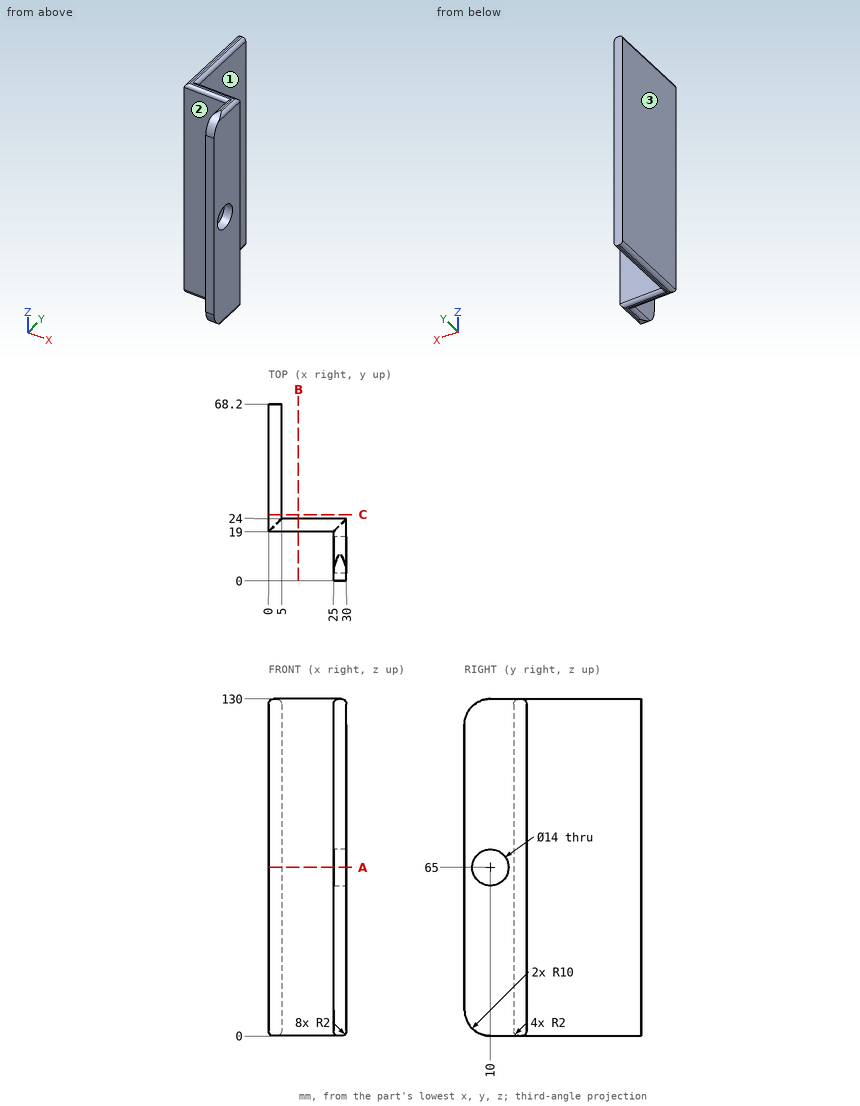
Verification items for this drawing (mm, ordinates from the low corner). A direction names the side the tool comes from. Coordinates: 2 decimals unless noted, no trailing zeros. Write each loop counter-clockwise with the first axis right and the second up, starting at its lowest first coordinate (ties: lowest second). Pieces come first, ordered by that corner, then holes. Notation, with made-up numbers: M -39,-40 L 3,-40 A13 ccw 3,-18 Z; hole C 53,37 d4. An arc over 180 degrees is marked long. Answer as a JSON object with one key per item and string values. Group by question number.
(1) Gauge pin test, flat ends, axial feed: pin 1 (12 mm diameter, centred on x = 9, z = 99.5, fed in from -Y); pin 2 (16 mm diameter, centred on y = 10, z = 65, fed in from -X); pin 3 (7.5 mm diameter, centred on x = 22, z = 80, fed in from +Y). Record the tip position at first contact, or that the pin passes through.
(2) Cross-section at C-C, the plane y = 25.5. Record the cut outline in (x, z), and give its area (3 significant figures).
(3) Tool access check on the marked faces 1, 2 and 3. Record the directions out of +Z, -Z, +X, -X, +Y, -Y that give a thin tool (end or side, any length) a straight path to the whole face; none if there is none.
(4) Material ranges on line 1 (Y direction, x = 28, z = 65); line 2 (Y direction, x = 29, z = 83.5); line 3 (Y direction, x = 7, z = 38.5), recorded low to high.
(5) Cross-section at B-B, the plane x = 11.5. Record the cut outline in (y, z).
(6) Cross-section at A-A, the plane z = 65. Record the cut outline in (x, y).
Reply:
{
 "1": {"pin 1": "y = 19", "pin 2": "x = 25", "pin 3": "y = 24"},
 "2": {"outline": "M 0,2 A2 ccw 2,0 L 3,0 A2 ccw 5,2 L 5,128 A2 ccw 3,130 L 2,130 A2 ccw 0,128 Z", "area": "647 mm²"},
 "3": {"face 1": "+Z, -Z, +X, +Y", "face 2": "+Z, -Z, -X, -Y", "face 3": "+Z, -Z, -X, +Y, -Y"},
 "4": {"line 1": "0 to 3, 17 to 24", "line 2": "0 to 24", "line 3": "19 to 24"},
 "5": {"outline": "M 19,2 A2 ccw 21,0 L 22,0 A2 ccw 24,2 L 24,128 A2 ccw 22,130 L 21,130 A2 ccw 19,128 Z"},
 "6": {"outline": "M 0,19 L 25,19 L 25,17 L 30,17 L 30,24 L 5,24 L 5,68.2 L 0,68.2 Z; M 25,0 L 30,0 L 30,3 L 25,3 Z"}
}
